Work out the finished part from the listing and answer in its coordinate system (mm). Face numbers are marked on the shaded views. A direction names the side the tool comes from. Give positions to 0.01 mm unless a question says otherwise; leave off trailing zeros. Order: outer loops, then holes, each group sorted by start corner. A loop starts at its lowest first (then second) coordinate and runs counter-clockwise, first axis right, second up. Notation, with made-up numbers: (62.25, -20.75) -> (66.25, -20.75) arc R22 cw to (66.25, -6.75) -> close; hole circle Ø10 at (-1, -11). An arc over 180 degrees is marked (long way). Answer as CSV lines item,"result". Start each with the question number.
1. A cutting plane is placed at C-C (y = 61). Give the vertices of the cut face in (x, z), then the cut area to 3 significant figures.
2. Flat-ended cylindrical pins translate along their axes: pin 1 (4.5 mm diameter, centred on x = -15, y = 6, fed in from +Z); pin 2 (2 mm diameter, centred on x = -5.5, y = 5, fed in from -Z); pin 3 (11 mm diameter, centred on x = -15, y = 6, fed in from -Z); pin 4 (2.5 mm diameter, centred on y = 61, z = 39.5, fed in from -X). Find the tip coordinate at first contact, or state that the pin passes through.
3. For the marked faces 5, 6, 7 and 8, determine the directions among +Z, -Z, +X, -X, +Y, -Y from which every point of the face is accessible in a straight line to the end or side of a thin tool.
4. For a pull along Y with two mould halves and no side action, classify the marked faces 1, 2, 3 and 4 as released by +Y, released by -Y, zero draft, split by the parting line, or undercut.
5. A cutting plane is placed at A-A (x = -10.25). Give the vertices of the cut face in (y, z).
6. Find the intervals of material crossed by L1, parallel to X at y = 6, z = 5.5; L2, parallel to Z at x = -0.75, y = 61; L3, parallel to Y at x = -13, z = 24, in increasing order.
7. A cutting plane is placed at D-D (y = 37). Give the vertices of the cut face in (x, z), then the cut area to 3 significant figures.
8. A cutting plane is placed at B-B (z = 8). Give the vertices of the cut face in (x, y), then the cut area to 3 significant figures.
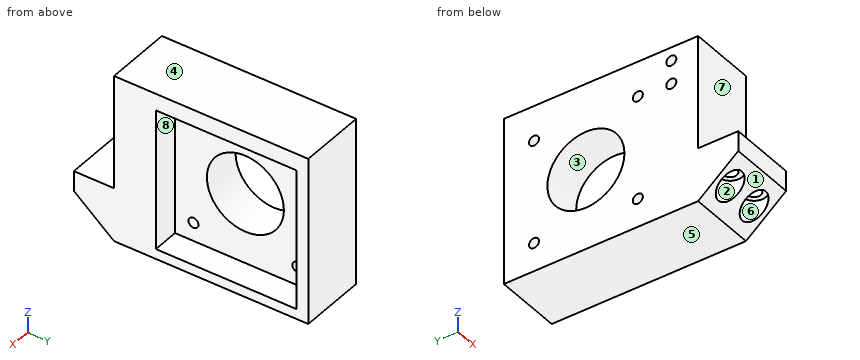
from build123d import *

# Parameters (mm, degrees)
SKETCH1_W           = 20
SKETCH1_H           = 50
BOSS_EXTRUDE1_DEPTH = 70
SKETCH2_R           = 1.5
SKETCH2_R_2         = 11.5
CUT_EXTRUDE2_DEPTH  = 60
SKETCH4_W           = 34
SKETCH4_H           = 12
CUT_EXTRUDE3_DEPTH  = 60
SKETCH8_R           = 2
CUT_EXTRUDE5_DEPTH  = 15
SKETCH9_W           = 42
SKETCH9_H           = 42
CUT_EXTRUDE6_DEPTH  = 8
CUT_EXTRUDE8_DEPTH  = 30
SKETCH17_R          = 3.5
CUT_EXTRUDE13_DEPTH = 9.18109305
SKETCH18_R          = 1.5
CUT_EXTRUDE14_DEPTH = 7


with BuildPart() as part:
    # Sketch1 → Boss-Extrude1 (new body)
    with BuildSketch(Plane(origin=(0, 0, 0), x_dir=(1, 0, 0), z_dir=(0, 1, 0))):
        with Locations((-10, -25)):
            Rectangle(SKETCH1_W, SKETCH1_H)
    extrude(amount=BOSS_EXTRUDE1_DEPTH)

    # Sketch2 → Cut-Extrude2 (cut)
    with BuildSketch(Plane(origin=(0, 0, 0), x_dir=(0, 0, -1), z_dir=(1, 0, 0))):
        with Locations((-8.5, 61)):
            Circle(SKETCH2_R)
        with Locations((-24, 45.5)):
            Circle(SKETCH2_R_2)
        with Locations((-8.5, 30)):
            Circle(SKETCH2_R)
        with Locations((-39.5, 30)):
            Circle(SKETCH2_R)
        with Locations((-39.5, 61)):
            Circle(SKETCH2_R)
    extrude(amount=-CUT_EXTRUDE2_DEPTH, mode=Mode.SUBTRACT)

    # Sketch4 → Cut-Extrude3 (cut)
    with BuildSketch(Plane(origin=(0, 0, 0), x_dir=(0, 0, -1), z_dir=(1, 0, 0))):
        with Locations((-33, 6)):
            Rectangle(SKETCH4_W, SKETCH4_H)
    extrude(amount=-CUT_EXTRUDE3_DEPTH, mode=Mode.SUBTRACT)

    # Sketch8 → Cut-Extrude5 (cut)
    with BuildSketch(Plane(origin=(0, 0, 0), x_dir=(-1, 0, 0), z_dir=(0, 0, -1))):
        with Locations((15, 6)):
            Circle(SKETCH8_R)
        with Locations((5, 6)):
            Circle(SKETCH8_R)
    extrude(amount=-CUT_EXTRUDE5_DEPTH, mode=Mode.SUBTRACT)

    # Sketch9 → Cut-Extrude6 (cut)
    with BuildSketch(Plane(origin=(0, 0, 0), x_dir=(0, 0, -1), z_dir=(1, 0, 0))):
        with Locations((-24, 45.5)):
            Rectangle(SKETCH9_W, SKETCH9_H)
    extrude(amount=-CUT_EXTRUDE6_DEPTH, mode=Mode.SUBTRACT)

    # Sketch11 → Cut-Extrude8 (cut)
    with BuildSketch(Plane(origin=(0, 0, 0), x_dir=(0, 0, -1), z_dir=(1, 0, 0))):
        Polygon((-10, 0), (0, 0), (0, 12), align=None)
    extrude(amount=-CUT_EXTRUDE8_DEPTH, mode=Mode.SUBTRACT)

    # Sketch17 → Cut-Extrude13 (cut)
    with BuildSketch(Plane(origin=(0, 0, 0), x_dir=(-1, 0, 0), z_dir=(0, 0, -1))):
        with Locations((15, 6)):
            Circle(SKETCH17_R)
        with Locations((5, 6)):
            Circle(SKETCH17_R)
    extrude(amount=-CUT_EXTRUDE13_DEPTH, mode=Mode.SUBTRACT)

    # Sketch18 → Cut-Extrude14 (cut)
    with BuildSketch(Plane.ZY.offset(20)):
        with Locations((46, 20)):
            Circle(SKETCH18_R)
        with Locations((39, 20)):
            Circle(SKETCH18_R)
    extrude(amount=-CUT_EXTRUDE14_DEPTH, mode=Mode.SUBTRACT)


solid = part.part
Answer sheet:
1,outline,"(-20, 0) -> (0, 0) -> (0, 3) -> (-8, 3) -> (-8, 7) -> (-20, 7) -> close; (-20, 10) -> (-8, 10) -> (-8, 38) -> (-20, 38) -> close; (-20, 41) -> (-8, 41) -> (-8, 45) -> (0, 45) -> (0, 50) -> (-20, 50) -> close"
1,area,"592 mm^2"
2,pin 1,"stops at z = 16"
2,pin 2,"stops at z = 9.18"
2,pin 3,"stops at z = 0.42"
2,pin 4,"passes through"
3,face 5,"-Z, +X, -X, +Y, -Y"
3,face 6,"-Z"
3,face 7,"+Z, +X, -X, -Y"
3,face 8,"+X"
4,face 1,"released by -Y"
4,face 2,"undercut"
4,face 3,"undercut"
4,face 4,"zero draft"
5,outline,"(0, 10) -> (12, 0) -> (70, 0) -> (70, 50) -> (12, 50) -> (12, 16) -> (0, 16) -> close; hole circle Ø3 at (30, 8.5); hole circle Ø3 at (30, 39.5); hole circle Ø23 at (45.5, 24); hole circle Ø3 at (61, 8.5); hole circle Ø3 at (61, 39.5)"
6,L1,"x = -20 to -18.5, -11.5 to -8.5, -1.5 to 0"
6,L2,"z = 0 to 3, 45 to 50"
6,L3,"y = 12 to 34, 57 to 70"
7,outline,"(-20, 0) -> (0, 0) -> (0, 3) -> (-8, 3) -> (-8, 16.25) -> (-20, 16.25) -> close; (-20, 31.75) -> (-8, 31.75) -> (-8, 45) -> (0, 45) -> (0, 50) -> (-20, 50) -> close"
7,area,"478 mm^2"
8,outline,"(-20, 2.4) -> (0, 2.4) -> (0, 24.5) -> (-8, 24.5) -> (-8, 28.59) -> (-20, 28.59) -> close; (-20, 31.41) -> (-8, 31.41) -> (-8, 59.59) -> (-20, 59.59) -> close; (-20, 62.41) -> (-8, 62.41) -> (-8, 66.5) -> (0, 66.5) -> (0, 70) -> (-20, 70) -> close; hole circle Ø7 at (-15, 6); hole circle Ø7 at (-5, 6)"
8,area,"871 mm^2"
